from build123d import *

# Parameters (mm, degrees)
F0_W     = 58
F0_H     = 44
F1_DEPTH = 7
F2_W     = 54
F2_H     = 40
F3_DEPTH = 5
F4_R     = 3.5
F5_DEPTH = 50
F6_R     = 3.5
F7_DEPTH = 60


with BuildPart() as f1:
    # F0 (on Top) → F1 (new body)
    with BuildSketch(Plane.XY):
        Rectangle(F0_W, F0_H)
    extrude(amount=F1_DEPTH)

    # F2 (on face) → F3 (cut)
    with BuildSketch(Plane.XY.offset(7)):
        Rectangle(F2_W, F2_H)
    extrude(amount=-F3_DEPTH, mode=Mode.SUBTRACT)

    # F4 (on face) → F5 (cut)
    with BuildSketch(Plane.XZ.offset(22)):
        with Locations((-15, 7)):
            Circle(F4_R)
        with Locations((-2, 7)):
            Circle(F4_R)
        with Locations((15, 7)):
            Circle(F4_R)
    extrude(amount=-F5_DEPTH, mode=Mode.SUBTRACT)

    # F6 (on face) → F7 (cut)
    with BuildSketch(Plane(origin=(-29, 0, 0), x_dir=(0, -1, 0), z_dir=(-1, 0, 0))):
        with Locations((0, 7)):
            Circle(F6_R)
    extrude(amount=-F7_DEPTH, mode=Mode.SUBTRACT)


solid = f1.part
The model under review builds one solid part; all positions refer to its coordinate system, in mm. A direction names the side the tool comes from. Give positions to 0.01 mm unless a question says otherwise; leave off trailing zeros. Write each loop counter-clockwise with the first axis right and the second up, starting at its lowest first coordinate (ties: lowest second). Pieces come first, ordered by that corner, then holes.
1. Add section A-A, the plane x = 25. Write out the cut boundary in (y, z).
2. Tool access review of faces 4 (the flat face through (0, 20, 3)), 5 (the flat face through (6, 21, 7)): name each direction out of +Z, -Z, +X, -X, +Y, -Y from which nothing blocks a thin tool from reaching the whole face with its end or side.
3. Draft analysis for pull direction X (two halves, no side actions). For faces 1 (the flat face through (6, -21, 7)), 2 (the flat face through (-29, 0, 3)), 3 (the cylindrical face through (-2.1, -21, 3.5)), state which applies: +X half, -X half, draft (parallel to the pull), parting line (faces both ways), or undercut.
4. For P1, Ø4, axis at x = 7.5, y = 13.5, coming from the -Z side; P2, Ø20, axis at x = -13, y = -0.5, coming from the +Z side, all flat-tipped, find the tip position at first contact; note any pin that passes through.
5. Add section B-B, the plane y = 0. Write out the cut boundary in (x, z).
6. Wall thickness on L1, parallel to X at y = 6, z = 4.5; L2, parallel to Y at x = -12, z = 2.75; L3, parallel to Z at x = -11, y = 18: over which ranges is each line inside the solid? List them lowest first.
Worked answers:
1. outline: (-22, 0) - (22, 0) - (22, 7) - (20, 7) - (20, 2) - (-20, 2) - (-20, 7) - (-22, 7) - close
2. face 4: +Z
2. face 5: +Z, +X, -X, +Y, -Y
3. face 1: draft
3. face 2: -X half
3. face 3: undercut
4. P1: stops at z = 0
4. P2: stops at z = 2
5. outline: (-29, 0) - (29, 0) - (29, 3.5) - (27, 3.5) - (27, 2) - (-27, 2) - (-27, 3.5) - (-29, 3.5) - close
6. L1: x = -29 to -27, 27 to 29
6. L2: y = -22 to -20, 20 to 22
6. L3: z = 0 to 2
